Model file for the job. Use its own axes, mm. Face numbers are marked on the shaded views. A direction names the side the tool comes from. Coordinates: 2 decimals unless noted, no trailing zeros. Order: outer loops, then holes, each group sorted by start corner. A loop starts at its lowest first (then second) coordinate and runs counter-clockwise, first axis right, second up. Notation, with made-up numbers: (-18, -21) -> (17, -21) arc R20 cw to (17, 12) -> close; hole circle Ø9 at (39.5, 7.25). An arc over 180 degrees is marked (long way). Return JSON: item names as keys, results as strings. Group by question number.
1) Cut at A-A (x = 11). Write the cut outline in (y, z), and give its area (3 significant figures).
2) Cut at D-D (y = 34). Write the cut outline in (x, z).
3) Probe line 1 (Y direction, x = 30, z = 2.75); line 2 (Z direction, x = 43, y = 20); line 3 (X direction, y = 21, z = 48.5). List the from-to ranges inside material, lowest first.
4) Pull direction X, two halves, no side cores. Call the marked faces 4, 5 and 6: +X half, -X half, draft (parallel to the pull), parting line (faces both ways), or undercut.
5) Which spindle directions (+Z, -Z, +X, -X, +Y, -Y) get a long thin tool onto all of the face, cutting with end or side? Do the marked faces 1, 2 and 3. Say none if no direction does.
6) Cut at B-B (y = 19). Write the cut outline in (x, z), and give its area (3 significant figures).
7) Flat gauge pins, fed straight in: pin 1 (15 mm diameter, centred on x = 40.5, y = 10, fed in from +Z); pin 2 (11 mm diameter, centred on y = 16, z = 42.5, fed in from +X); pin 3 (10 mm diameter, centred on y = 25, z = 5.5, fed in from +X). Where does each tip first touch, or does it go through?
8) Cut at C-C (x = 18.5). Write the cut outline in (y, z).
Autodesk Fusion 360 part; units mm, degrees
sketch "Sketch2" plane through (0, 0, 0) normal (0, 1, 0) x (1, 0, 0)
  line L0 (0, -10) -> (0, -50.06)
  line L1 (0, -50.06) -> (30, -50.06)
  line L2 (30, -50.06) -> (30, -40.06)
  line L3 (10, 0) -> (50, 0)
  line L4 (50, 0) -> (50, -10)
  arc A0 (10, 0) -> (0, -10) centre (10, -10) ccw
  line L5 (50, -10) -> (20, -10)
  line L6 (30, -40.06) -> (10, -40.06)
  line L7 (10, -40.06) -> (10, -20)
  arc A1 (20, -10) -> (10, -20) centre (20, -20) ccw
  point P0 (10, -10)
  dimension "d9" = 50.06
  dimension "d10" = 30
  dimension "d11" = 10
  dimension "d12" = 50
  dimension "d13" = 10
  dimension "d14" = 10
  dimension "d15" = 40
  dimension "d16" = 20
  dimension "d17" = 10
extrude "Extrude1" add sketch "Sketch2" along normal blind 40
sketch "Sketch5" plane through (0, 0, 50.06) normal (0, 0, 1) x (-1, 0, 0)
  line L0 (0, 0) -> (-30, 0)
  line L1 (-30, 0) -> (-30, -40)
  line L2 (-30, -40) -> (0, -40)
  line L3 (0, -40) -> (0, 0)
  line L4 (0, 0) -> (-20, 0)
  line L5 (-30, -10) -> (-30, -30)
  line L6 (-20, -40) -> (0, -40)
  line L7 (0, -40) -> (0, 0)
  arc A0 (-30, -30) -> (-20, -40) centre (-20, -30) ccw
  arc A1 (-20, 0) -> (-30, -10) centre (-20, -10) ccw
  dimension "d24" = 10
  dimension "d25" = 10
extrude "Extrude2" cut sketch "Sketch5" against normal blind 10 contours L0 L1 A1
extrude "Extrude3" cut sketch "Sketch5" against normal blind 10 contours L1 L2 A0
sketch "Sketch6" plane through (0, 0, 10) normal (0, 0, 1) x (-1, 0, 0)
  line L0 (-20, 0) -> (-50, 0)
  line L1 (-50, 0) -> (-50, -40)
  line L2 (-50, -40) -> (-20, -40)
  line L3 (-20, -40) -> (-20, 0)
  line L4 (-20, 0) -> (-30, 0)
  circle A0 centre (-30, -20) radius 10
  circle A1 centre (-30, -20) radius 20
  dimension "d30" = 10
extrude "Extrude4" cut sketch "Sketch6" against normal blind 10 contours A0
extrude "Extrude5" cut sketch "Sketch6" against normal blind 10 contours L0 L1 A1
extrude "Extrude6" cut sketch "Sketch6" against normal blind 10 contours L1 L2 A1
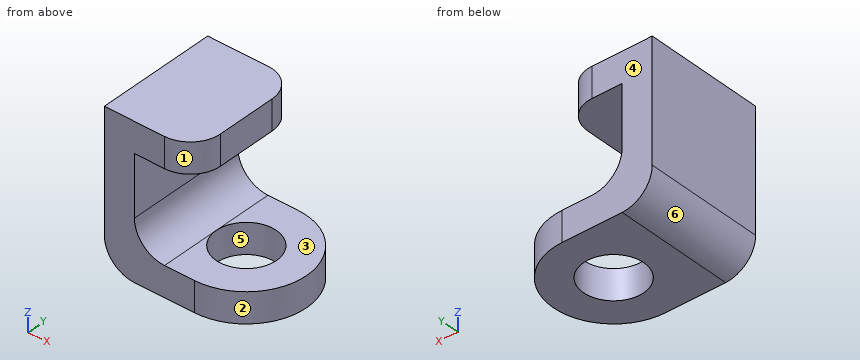
Answers below:
{
 "1": {"outline": "(0, 0) -> (40, 0) -> (40, 15.64) -> (0, 15.64) -> close; (0, 40.06) -> (40, 40.06) -> (40, 50.06) -> (0, 50.06) -> close", "area": "1,030 mm^2"},
 "2": {"outline": "(0, 10) arc R10 ccw to (10, 0) -> (44.28, 0) -> (44.28, 10) -> (20, 10) arc R10 cw to (10, 20) -> (10, 40.06) -> (29.17, 40.06) -> (29.17, 50.06) -> (0, 50.06) -> close"},
 "3": {"line 1": "y = 0 to 10, 30 to 40", "line 2": "z = 0 to 10", "line 3": "x = 0 to 30"},
 "4": {"face 4": "draft", "face 5": "undercut", "face 6": "-X half"},
 "5": {"face 1": "+Z, +X, -Y", "face 2": "+Z, -Z, +X", "face 3": "+X, +Y, -Y"},
 "6": {"outline": "(0, 10) arc R10 ccw to (10, 0) -> (20.05, 0) -> (20.05, 10) -> (20, 10) arc R10 cw to (10, 20) -> (10, 40.06) -> (30, 40.06) -> (30, 50.06) -> (0, 50.06) -> close; (39.95, 0) -> (49.97, 0) -> (49.97, 10) -> (39.95, 10) -> close", "area": "901 mm^2"},
 "7": {"pin 1": "stops at z = 10", "pin 2": "stops at x = 30", "pin 3": "stops at x = 50"},
 "8": {"outline": "(0, 0) -> (40, 0) -> (40, 10.11) -> (0, 10.11) -> close; (0, 40.06) -> (40, 40.06) -> (40, 50.06) -> (0, 50.06) -> close"}
}
